from build123d import *

# Parameters (mm, degrees)
SKETCH_1_R          = 1.6
EXTRUDE_1_DEPTH     = 3
CUT_EXTRUDE_START   = -3
SKETCH_2_R          = 1.6
CUT_EXTRUDE_1_DEPTH = 3
CUT_EXTRUDE_2_DEPTH = 3


with BuildPart() as part:
    # 草图1 → 凸台-拉伸1 (new body)
    with BuildSketch(Plane(origin=(0, 0, 0), x_dir=(1, 0, 0), z_dir=(0, 1, 0))):
        with BuildLine():
            Line((-32, 30), (32, 30))
            ThreePointArc((32, 30), (34.121320344, 29.121320344), (35, 27))
            Line((35, 27), (35, -27))
            ThreePointArc((35, -27), (34.121320344, -29.121320344), (32, -30))
            Line((32, -30), (-32, -30))
            ThreePointArc((-32, -30), (-34.121320344, -29.121320344), (-35, -27))
            Line((-35, -27), (-35, 27))
            ThreePointArc((-35, 27), (-34.121320344, 29.121320344), (-32, 30))
        make_face()
        with Locations(Location((-32, 27, 0), (0, 0, 270))):
            Circle(SKETCH_1_R, mode=Mode.SUBTRACT)
        with Locations(Location((32, 27, 0), (0, 0, 270))):
            Circle(SKETCH_1_R, mode=Mode.SUBTRACT)
        with Locations(Location((-32, -27, 0), (0, 0, 270))):
            Circle(SKETCH_1_R, mode=Mode.SUBTRACT)
        with Locations(Location((32, -27, 0), (0, 0, 270))):
            Circle(SKETCH_1_R, mode=Mode.SUBTRACT)
    extrude(amount=EXTRUDE_1_DEPTH)

    # 草图2 → 切除-拉伸1 (cut)
    with BuildSketch(Plane(origin=(0, 3, 0), x_dir=(1, 0, 0), z_dir=(0, 1, 0)).offset(CUT_EXTRUDE_START)):
        with Locations(Location((-27, 11, 0), (0, 0, 270))):
            Circle(SKETCH_2_R)
        with Locations(Location((27, 11, 0), (0, 0, 90))):
            Circle(SKETCH_2_R)
        with Locations(Location((-32, 27, 0), (0, 0, 270))):
            Circle(SKETCH_2_R)
    extrude(amount=CUT_EXTRUDE_1_DEPTH, mode=Mode.SUBTRACT)

    # 草图3 → 切除-拉伸2 (cut)
    with BuildSketch(Plane.XZ):
        with BuildLine():
            Line((-22, 20), (-5, 20))
            ThreePointArc((-5, 20), (-2.878679656, 19.121320344), (-2, 17))
            Line((-2, 17), (-2, 12))
            ThreePointArc((-2, 12), (-2.878679656, 9.878679656), (-5, 9))
            Line((-5, 9), (-22, 9))
            ThreePointArc((-22, 9), (-24.121320344, 9.878679656), (-25, 12))
            Line((-25, 12), (-25, 17))
            ThreePointArc((-25, 17), (-24.121320344, 19.121320344), (-22, 20))
        make_face()
        with BuildLine():
            Line((-22, -6), (-20, -6))
            ThreePointArc((-20, -6), (-17.878679656, -6.878679656), (-17, -9))
            Line((-17, -9), (-17, -17))
            ThreePointArc((-17, -17), (-16.121320344, -19.121320344), (-14, -20))
            Line((-14, -20), (-5, -20))
            ThreePointArc((-5, -20), (-2.878679656, -19.121320344), (-2, -17))
            Line((-2, -17), (-2, 2))
            ThreePointArc((-2, 2), (-2.878679656, 4.121320344), (-5, 5))
            Line((-5, 5), (-22, 5))
            ThreePointArc((-22, 5), (-24.121320344, 4.121320344), (-25, 2))
            Line((-25, 2), (-25, -3))
            ThreePointArc((-25, -3), (-24.121320344, -5.121320344), (-22, -6))
        make_face()
        with BuildLine():
            Line((25, 17), (25, 12))
            ThreePointArc((25, 12), (24.121320344, 9.878679656), (22, 9))
            Line((22, 9), (5, 9))
            ThreePointArc((5, 9), (2.878679656, 9.878679656), (2, 12))
            Line((2, 12), (2, 17))
            ThreePointArc((2, 17), (2.878679656, 19.121320344), (5, 20))
            Line((5, 20), (22, 20))
            ThreePointArc((22, 20), (24.121320344, 19.121320344), (25, 17))
        make_face()
        with BuildLine():
            Line((17, -9), (17, -17))
            ThreePointArc((17, -17), (16.121320344, -19.121320344), (14, -20))
            Line((14, -20), (4.999263136, -19.997789228))
            ThreePointArc((4.999263136, -19.997789228), (2.878419152, -19.118849125), (2, -16.997789318))
            Line((2, -16.997789318), (2, 2))
            ThreePointArc((2, 2), (2.878679656, 4.121320344), (5, 5))
            Line((5, 5), (22, 5))
            ThreePointArc((22, 5), (24.121320344, 4.121320344), (25, 2))
            Line((25, 2), (25, -3))
            ThreePointArc((25, -3), (24.121320344, -5.121320344), (22, -6))
            Line((22, -6), (20, -6))
            ThreePointArc((20, -6), (17.878679656, -6.878679656), (17, -9))
        make_face()
    extrude(amount=-CUT_EXTRUDE_2_DEPTH, mode=Mode.SUBTRACT)


solid = part.part
Here's how the part is built. I have some questions about the finished solid (model axes, mm). A direction names the side the tool comes from. Coordinates: 2 decimals unless noted, no trailing zeros. Loops run counter-clockwise (first coordinate to the right, second up) from the corner with the lowest first, then second, coordinate; pieces in that order, holes last. Notation, with made-up numbers: (17, 47.5) -> (30, 47.5) arc R17 ccw to (30, 60.5) -> close; hole circle Ø1 at (30, -7). An arc over 180 degrees is marked (long way). Use one line per item in the form item = value. Start each with the question number.
(1) If we section it at D-D (x = -24): Please give me the cut outline in (y, z), then the cut area to 3 significant figures.
(2) Please list where these lines run through material, in increasing order: line 1 along X through (y, z) = (1.4, 0.5); line 2 along X through (y, z) = (0.8, -11); line 3 along X through (y, z) = (1.6, -13.5).
(3) We'd pull the mould along Z, two halves only. Please class faces 1 (the face through (34.1, 1.48, -29.14)), 2 (the face through (17.9, 1.48, -6.86)), 3 (the face through (-24.14, 1.48, -5.1)), 4 (the face through (-34.1, 1.48, 29.14)): pulls with the +Z half, pulls with the -Z half, needs draft (parallel to the pull), parting line crosses it, or undercut.
(4) On a 3-axis mill with a long thin cutter (end or side, diameter ignored), from which of +Z, -Z, +X, -X, +Y, -Y can I reach the whole of each face in a straight line? I mean faces 5 (the face through (0, 3, 0)), 6 (the face through (-25, 1, 0)). Say none if no direction works.
(5) If we section it at A-A (x = -6): Please give me the cut outline in (y, z).
(6) If we section it at C-C (z = -11): Please give me the cut outline in (x, y).
(7) Will these pins go through, and if not, where does the flat tip stop? pin 1 (1.9 mm diameter, centred on x = -32, z = 27, fed in from -Y); pin 2 (4 mm diameter, centred on x = 27, z = -11, fed in from -Y).
(8) If we section it at B-B (x = 27): Please give me the cut outline in (y, z).
Verdict:
q1.outline = (0, -30) -> (3, -30) -> (3, -5.24) -> (0, -5.24) -> close; (0, 4.24) -> (3, 4.24) -> (3, 9.76) -> (0, 9.76) -> close; (0, 19.24) -> (3, 19.24) -> (3, 30) -> (0, 30) -> close
q1.area = 123 mm²
q2.line_1 = -35 to -25, -2 to 2, 25 to 35
q2.line_2 = -35 to -28.6, -25.4 to -17, -2 to 2, 17 to 25.4, 28.6 to 35
q2.line_3 = -35 to -17, -2 to 2, 17 to 35
q3.face_1 = pulls with the -Z half
q3.face_2 = undercut
q3.face_3 = undercut
q3.face_4 = pulls with the +Z half
q4.face_5 = +Z, -Z, +X, -X, +Y
q4.face_6 = +Y, -Y
q5.outline = (0, -30) -> (3, -30) -> (3, -20) -> (0, -20) -> close; (0, 5) -> (3, 5) -> (3, 9) -> (0, 9) -> close; (0, 20) -> (3, 20) -> (3, 30) -> (0, 30) -> close
q6.outline = (-35, 0) -> (-28.6, 0) -> (-28.6, 3) -> (-35, 3) -> close; (-25.4, 0) -> (-17, 0) -> (-17, 3) -> (-25.4, 3) -> close; (-2, 0) -> (2, 0) -> (2, 3) -> (-2, 3) -> close; (17, 0) -> (25.4, 0) -> (25.4, 3) -> (17, 3) -> close; (28.6, 0) -> (35, 0) -> (35, 3) -> (28.6, 3) -> close
q7.pin_1 = through
q7.pin_2 = 0
q8.outline = (0, -30) -> (3, -30) -> (3, -12.6) -> (0, -12.6) -> close; (0, -9.4) -> (3, -9.4) -> (3, 30) -> (0, 30) -> close
